Here's how the part is built. I have some questions about the finished solid (model axes, mm). A direction names the side the tool comes from. Coordinates: 2 decimals unless noted, no trailing zeros. Order: outer loops, then holes, each group sorted by start corner. A loop starts at its lowest first (then second) coordinate and runs counter-clockwise, first axis right, second up. Notation, with made-up numbers: (52.5, 71) - (59.5, 71) arc R23 cw to (59.5, 83) - close; hole circle Ø5 at (20, 8.25). An arc over 180 degrees is marked (long way). Answer in a Markdown table with one row per item. Add a question column.
Item 1: Thinking about a two-plate mould opening in X: for faces 1 (the cylindrical face through (33.5, 2.38, -113.42)), 2 (the flat face through (1, 17.526, -77)), 3 (the flat face through (45.4, 2.4, -63.5)), which applies, +X half, -X half, draft (parallel to the pull), parting line (faces both ways), or undercut?
Item 2: On a 3-axis mill with a long thin cutter (end or side, diameter ignored), from which of +Z, -Z, +X, -X, +Y, -Y can I reach the whole of each face in a straight line? I mean faces 4 (the cylindrical face through (47.31, 11.09, -100.78)), 5 (the flat face through (51, 2, -77.005)), 6 (the flat face through (16, 17.526, -50)). Say none if no direction works.
Item 3: I want a section at C-C (y = 1.75). Please give me the cut outline in (x, z) (1 decimal).
Item 4: I want a section at B-B (x = 25.5). Please give me the cut outline in (y, z).
Item 5: I want a section at A-A (z = -97.5). Please give me the cut outline in (x, y), plus the area to 3 significant figures.
Item 6: If I drill on line 1 along Z through (x, y) = (47.5, 12.5); line 2 along Z through (x, y) = (46, 1); line 3 along X through (y, z) = (2.75, -86.5), over which ranges is the centre line in solid material (lowest first)? Write a range as from..to.
Item 7: I want a section at D-D (y = 7.5). Count the separate pieces of the cut face and the enclosed holes in it, plus the area to 3 significant figures.
Item 8: Will these pins go through, and if not, where does the flat tip stop? pin 1 Ø4 at (y, z) = (3, -97) entering from +X; pin 2 Ø4 at (x, y) = (5, 4.5) entering from -Z; pin 3 Ø6 at (x, z) = (4.5, -83.5) entering from +Y.
```python
from build123d import *

# Parameters (mm, degrees)
SKETCH1_R         = 36.449
SKETCH1_R_2       = 4.7625
EXTRUDE1_DEPTH    = 4.826
SKETCH2_R         = 3.175
EXTRUDE2_DEPTH    = 12.7
CIRPATTERN1_COUNT = 12
EXTRUDE3_DEPTH    = 19.05
CIRPATTERN2_COUNT = 4


with BuildPart() as part:
    # Sketch1 → Extrude1 (new body)
    with BuildSketch(Plane(origin=(0, 0, 0), x_dir=(1, 0, 0), z_dir=(0, 1, 0))):
        with Locations(Location((31.896411717, 77.004913135, 0), (0, 0, 270))):  # turned: the seam where the file's is
            Circle(SKETCH1_R)
        with Locations(Location((31.896411717, 77.004913135, 0), (0, 0, 270))):  # turned: the seam where the file's is
            Circle(SKETCH1_R_2, mode=Mode.SUBTRACT)
    extrude(amount=EXTRUDE1_DEPTH)

    # Sketch2 → Extrude2 (add)
    with BuildSketch(Plane(origin=(0, 4.826, 0), x_dir=(1, 0, 0), z_dir=(0, 1, 0))):
        with Locations(Location((63.011411717, 77.004913135, 0), (0, 0, 270))):  # turned: the seam where the file's is
            Circle(SKETCH2_R)
    extrude2 = extrude(amount=EXTRUDE2_DEPTH)

    # CirPattern1: Extrude2 ×12 about axis
    cirpattern1_axis = Axis((31.896411717, 0, -77.004913135), (0, 1, 0))
    for i in range(1, CIRPATTERN1_COUNT):
        add(extrude2.rotate(cirpattern1_axis, i * 360 / CIRPATTERN1_COUNT))

    # Sketch3 → Extrude3 (cut)
    with BuildSketch(Plane(origin=(0, 4.826, 0), x_dir=(1, 0, 0), z_dir=(0, 1, 0))):
        with BuildLine():
            Line((31.896411717, 89.62444152), (31.896411717, 102.416748175))
            ThreePointArc((31.896411717, 102.416748175), (41.621099973, 100.482387412), (49.865292596, 94.973794014))
            Line((49.865292596, 94.973794014), (40.819765813, 85.928267231))
            ThreePointArc((40.819765813, 85.928267231), (36.725696154, 88.66383712), (31.896411717, 89.62444152))
        make_face()
    extrude3 = extrude(amount=-EXTRUDE3_DEPTH, mode=Mode.SUBTRACT)

    # CirPattern2: Extrude3 ×4 about axis
    cirpattern2_axis = Axis((31.896411717, 4.826, -77.004913135), (0, 1, 0))
    for i in range(1, CIRPATTERN2_COUNT):
        add(extrude3.rotate(cirpattern2_axis, i * 360 / CIRPATTERN2_COUNT), mode=Mode.SUBTRACT)


solid = part.part
```
Values follow:
| question | item | result |
|---|---|---|
| 1 | face 1 | parting line |
| 1 | face 2 | draft |
| 1 | face 3 | undercut |
| 2 | face 4 | +Y |
| 2 | face 5 | +Y, -Y |
| 2 | face 6 | +Z, -Z, +X, -X, +Y |
| 3 | outline | circle Ø72.9 at (31.9, -77); hole (6.5, -77) arc R25.4 ccw to (13.9, -95) - (23, -85.9) arc R12.6 cw to (19.3, -77) - close; hole (13.9, -59) - (23, -68.1) arc R12.6 cw to (31.9, -64.4) - (31.9, -51.6) arc R25.4 ccw to start; hole circle Ø9.5 at (31.9, -77); hole (31.9, -102.4) arc R25.4 ccw to (49.9, -95) - (40.8, -85.9) arc R12.6 cw to (31.9, -89.6) - close; hole (40.8, -68.1) arc R12.6 cw to (44.5, -77) - (57.3, -77) arc R25.4 ccw to (49.9, -59) - close |
| 4 | outline | (0, -112.89) - (4.83, -112.89) - (4.83, -66.13) - (0, -66.13) - close; (0, -52.41) - (4.83, -52.41) - (4.83, -41.12) - (0, -41.12) - close |
| 5 | outline | (1.76, 0) - (31.9, 0) - (31.9, 4.83) - (1.76, 4.83) - close; (46.92, 0) - (62.04, 0) - (62.04, 4.83) - (46.92, 4.83) - close |
| 5 | area | 218 mm^2 |
| 6 | line 1 | z = -107.13..-100.78, -53.23..-46.88 |
| 6 | line 2 | z = -110.61..-98.14, -91.11..-77, -62.9..-43.4 |
| 6 | line 3 | x = -3.29..8.33, 22.4..40.21, 41.39..67.09 |
| 7 | separate pieces | 12 |
| 7 | enclosed holes | 0 |
| 7 | area | 380 mm^2 |
| 8 | pin 1 | stops at x = 63.59 |
| 8 | pin 2 | stops at z = -103.63 |
| 8 | pin 3 | stops at y = 4.83 |
